```python
from build123d import *

# Parameters (mm, degrees)
SKETCH019_W             = 81
SKETCH019_H             = 26
SKETCH019_W_2           = 77
SKETCH019_H_2           = 22
REVOLUTION_ANGLE        = 35
SKETCH020_W             = 81
SKETCH020_H             = 26
SKETCH020_W_2           = 77
SKETCH020_H_2           = 22
PAD010_DEPTH            = 60
POCKET006_DEPTH         = 81.001
SKETCH022_W             = 81
SKETCH022_H             = 26
SKETCH022_W_2           = 77
SKETCH022_H_2           = 22
PAD011_DEPTH            = 15
CHAMFER002_SIZE         = 1
BODY005_PLACEMENT_ANGLE = 180


with BuildPart() as part:
    # Sketch019 → Revolution (revolve)
    with BuildSketch(Plane(origin=(310, 157, 2), x_dir=(0, 1, 0), z_dir=(1, 0, 0))):
        with Locations((40.5, 13)):
            Rectangle(SKETCH019_W, SKETCH019_H)
        with Locations((40.5, 13)):
            Rectangle(SKETCH019_W_2, SKETCH019_H_2, mode=Mode.SUBTRACT)
    revolve(axis=Axis((310, 157, 2), (0, 1, 0)), revolution_arc=REVOLUTION_ANGLE)

    # Sketch020 (on Face9 of Revolution) → Pad010 (new body)
    with BuildSketch(Plane(origin=(207.07343, 0, -144.994376), x_dir=(0, 1, 0), z_dir=(0.819152, 0, -0.573576))):
        with Locations((197.5, 192.446999)):
            Rectangle(SKETCH020_W, SKETCH020_H)
        with Locations((197.5, 192.446999)):
            Rectangle(SKETCH020_W_2, SKETCH020_H_2, mode=Mode.SUBTRACT)
    extrude(amount=PAD010_DEPTH)

    # Sketch021 (on Face11 of Pad010) → Pocket006 (cut, through all)
    with BuildSketch(Plane(origin=(0, 157, 0), x_dir=(0, 0, -1), z_dir=(0, -1, 0))):
        Polygon((21.76561, 366.605616), (32.414586, 359.149123), (24.958093, 348.500146), align=None)
    extrude(amount=-POCKET006_DEPTH, mode=Mode.SUBTRACT)

    # Sketch022 (on Face4 of Pocket006) → Pad011 (join)
    with BuildSketch(Plane(origin=(310, 0, 0), x_dir=(0, 1, 0), z_dir=(-1, 0, 0))):
        with Locations((197.5, -15)):
            Rectangle(SKETCH022_W, SKETCH022_H)
        with Locations((197.5, -15)):
            Rectangle(SKETCH022_W_2, SKETCH022_H_2, mode=Mode.SUBTRACT)
    extrude(amount=PAD011_DEPTH)

    # Chamfer002
    chamfer002_edges = [part.edges().sort_by_distance(p)[0] for p in [
        (302.5, 159, 4),
        (295, 197.5, 4),
        (295, 159, 15),
        (302.5, 159, 26),
        (295, 197.5, 26),
        (295, 236, 15),
        (302.5, 236, 26),
        (317.216939, 236, 24.889207),
        (317.216939, 159, 24.889207),
        (310.601412, 159, 3.907434),
        (331.216378, 159, -10.414319),
        (310.601412, 236, 3.907434),
        (331.216378, 236, -10.414319),
        (348.340396, 236, 4.452356),
        (348.340396, 159, 4.452356),
    ]]
    chamfer(chamfer002_edges, length=CHAMFER002_SIZE)


with BuildPart() as part_1:
    # Body005 placement: moved
    add(part.part.moved(Location((0, 395, 30))).rotate(Axis((0, 395, 30), (1, 0, 0)), BODY005_PLACEMENT_ANGLE))


solid = part_1.part
```
Part model, mm, in its own coordinate system. A direction names the side the tool comes from. Round coordinates to 2 decimals unless told otherwise and drop trailing zeros. Order: outer loops, then holes, each group sorted by start corner. A loop starts at its lowest first (then second) coordinate and runs counter-clockwise, first axis right, second up. Notation, with made-up numbers: M 68,36.5 L 83,36.5 A10 ccw 83,40.5 Z; hole C 18.25,51 d4. An arc over 180 degrees is marked long. Answer in a Markdown table with one row per item. Add a question column.
Q1. Mould opens along Z. For faces 1 (the face through (317.71, 196.93, 3.17)), 2 (the face through (295.4, 159.2, 25.8)), 3 (the face through (335, 238, 28)) say: +Z half, -Z half, draft (parallel to the pull), parting line (faces both ways), or undercut.
Q2. Cut at A-A on x = 303.5. Give the cut face in (y, z), and give its area (3 significant figures).
Q3. Wall check: L1, parallel to Y at x = 332.5, z = 24.5; L2, parallel to Z at x = 324, y = 229.5; L3, parallel to Z at x = 314, y = 195. Give the ranges that are in metal, low to high. Write a range as from..to.
Q4. Cut at C-C on z = 23.5. Give the cut face in (x, y).
Q5. Cut at B-B on y = 215.5. Give the cut face in (x, z), and give its area (3 significant figures).
Q6. 3-axis set-ups, long thin cutter, end or side, ignore diameter. For faces 4 (the face through (332.195, 159.507, 40.498)), 5 (the face through (295.4, 235.8, 4.2)), 6 (the face through (349.143, 198.067, 23.668)): which of +Z, -Z, +X, -X, +Y, -Y reach the whole face in a straight line?
Q7. Cut at D-D on z = 34.5. Give the cut face in (x, y), and give its area (3 significant figures).
Q8. Pin check, flat tips, straight feed: pin 1 (2 mm diameter, centred on x = 305.5, y = 184, fed in from +Z); pin 2 (10 mm diameter, centred on x = 313, y = 222, fed in from +Z); pin 3 (12 mm diameter, centred on x = 305, y = 203.5, fed in from +Z); pin 4 (2 mm diameter, centred on x = 364, z = 33.5, fed in from -Y). Stop position of each tip, or through.
Established:
| question | item | result |
|---|---|---|
| 1 | face 1 | -Z half |
| 1 | face 2 | undercut |
| 1 | face 3 | draft |
| 2 | outline | M 157,2 L 238,2 L 238,28 L 157,28 Z; hole M 159,5 L 160,4 L 235,4 L 236,5 L 236,25 L 235,26 L 160,26 L 159,25 Z |
| 2 | area | 414 mm2 |
| 3 | L1 | y = 157..159, 236..238 |
| 3 | L2 | z = 6.09..8.5, 35.36..37.8 |
| 3 | L3 | z = 2.31..4.34, 28.36..30.8 |
| 4 | outline | M 295,157 L 348.9,157 L 348.9,238 L 295,238 L 295,237 L 296,236 L 343.67,236 L 345.42,235 L 345.42,160 L 343.67,159 L 296,159 L 295,158 Z |
| 5 | outline | M 295,2 L 310,2 A26 ccw 324.91,6.7 L 374.06,41.12 L 372.91,42.75 L 323.77,8.34 A24 cw 310,4 L 296,4 L 295,3 Z; M 295,27 L 296,26 L 310,26 A2 ccw 311.15,26.36 L 351.29,54.47 L 348.5,54.96 L 310,28 L 295,28 Z |
| 5 | area | 307 mm2 |
| 6 | face 4 | none |
| 6 | face 5 | -X |
| 6 | face 6 | -Z, +X, +Y, -Y |
| 7 | outline | M 319.28,157 L 364.61,157 L 364.61,238 L 319.28,238 Z; hole M 322.77,160 L 324.51,159 L 359.38,159 L 361.13,160 L 361.13,235 L 359.38,236 L 324.51,236 L 322.77,235 Z |
| 7 | area | 722 mm2 |
| 8 | pin 1 | stops at z = 28 |
| 8 | pin 2 | stops at z = 33.6 |
| 8 | pin 3 | stops at z = 28.7 |
| 8 | pin 4 | stops at y = 157 |
